Here's the drawing with two shaded views (mm, measured from the low corner). I have some questions. Round coordinates to 2 decimals unless told otherwise and drop trailing zeros. Order: outer loops, then holes, each group sorted by start corner. A loop starts at its lowest first (then second) coordinate and runs counter-clockwise, first axis right, second up. Notation, with made-up numbers: (83.5, 82) -> (116.5, 82) arc R21 cw to (116.5, 113) -> close; hole circle Ø4 at (87.5, 53.5). An arc over 180 degrees is marked (long way). One line per question, with ' | ' between items.
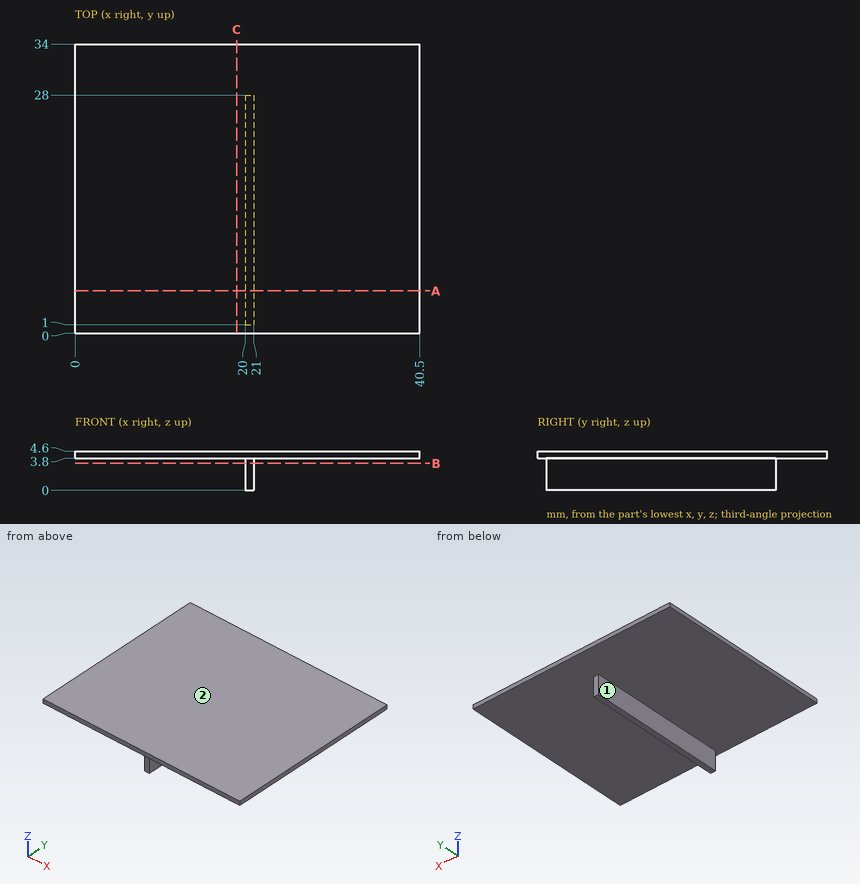
1. I want a section at B-B on z = 3.2. List the corners of the cut face in (x, y) for me, and give its area (3 significant figures).
From the geometry:
outline: (20, 1) -> (21, 1) -> (21, 28) -> (20, 28) -> close | area: 27.0 mm²
2. I need wall thicknesses on probe 1 along X at (y, z) = (17.5, 3.25); probe 2 along Z at (x, y) = (38, 10). Which ranges of each line are inside material? Lowest first, please.
From the geometry:
probe 1: x = 20 to 21 | probe 2: z = 3.8 to 4.6
3. I want a section at A-A on y = 5. List the corners of the cut face in (x, z) for me, and give its area (3 significant figures).
From the geometry:
outline: (0, 3.8) -> (20, 3.8) -> (20, 0) -> (21, 0) -> (21, 3.8) -> (40.5, 3.8) -> (40.5, 4.6) -> (0, 4.6) -> close | area: 36.2 mm²
4. I want a section at C-C on x = 19. List the corners of the cut face in (y, z) for me.
From the geometry:
outline: (0, 3.8) -> (34, 3.8) -> (34, 4.6) -> (0, 4.6) -> close
5. I'm going to push flat-ended pins straight in: pin 1 (0.8 mm diameter, centred on x = 20.5, z = 2.5, fed in from +Y); pin 2 (1.5 mm diameter, centred on x = 21, z = 2, fed in from -Y); pin 3 (12 mm diameter, centred on x = 6, y = 21.5, fed in from -Z). Where does each tip first touch, or does it pass through?
From the geometry:
pin 1: stops at y = 28 | pin 2: stops at y = 1 | pin 3: stops at z = 3.8
6. If we mould it in two halves opening along Z, with no side actions, what happens to the marked faces 1 and 2? For each: pulls with the +Z half, pulls with the -Z half, needs draft (parallel to the pull), parting line crosses it, or undercut.
From the geometry:
face 1: needs draft | face 2: pulls with the +Z half
